Design review of the part shown in the three views and the two pictorial views. Dimensions are in mm from the part's minimum x, y and z. Round coordinates to 2 decimals unless told otherwise and drop trailing zeros. Loops run counter-clockwise (first coordinate to the right, second up) from the corner with the lowest first, then second, coordinate; pieces in that order, holes last.
1. Clearance check with flat-ended pins moving along their axes: pin 1 Ø0.7 at (y, z) = (31.5, 1) entering from -X; pin 2 Ø1.2 at (x, z) = (9.5, 0.5) entering from +Y; pin 3 Ø0.7 at (y, z) = (33, 1.5) entering from +X. State where each tip first meets the part, or that it passes through.
2. To check wall thickness, follow line 1 along X through (y, z) = (32.2, 0.75); line 2 along Y through (x, z) = (19.7, 1); line 3 along X through (y, z) = (27, 1.4). State the ranges of each line that lie inside material, in increasing order.
3. Consider section D-D on x = 6. State the section outline as (y, z) points, then the cut area to 3 significant figures.
4. Consider section B-B on y = 32.2. State the section outline as (x, z) points, then the cut area to 3 significant figures.
5. Consider section C-C on x = 19.7. State the section outline as (y, z) points.
6. Consider section A-A on z = 1.6. State the section outline as (x, y) points.
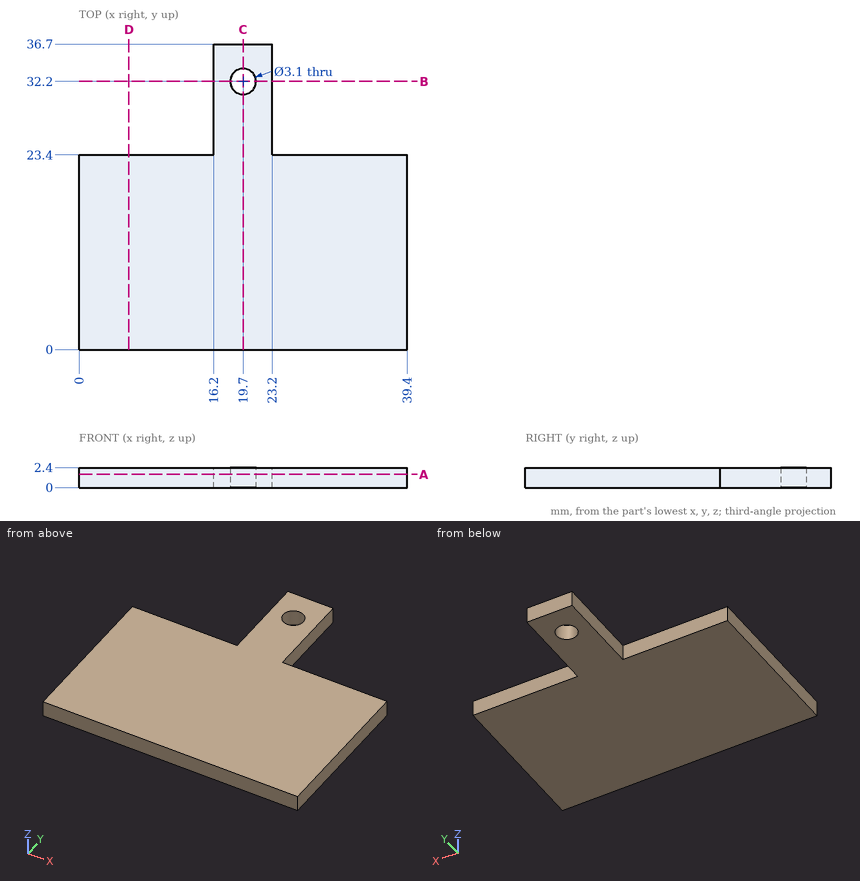
Resolved:
1. pin 1: stops at x = 16.2
1. pin 2: stops at y = 23.4
1. pin 3: stops at x = 23.2
2. line 1: x = 16.2 to 18.15, 21.25 to 23.2
2. line 2: y = 0 to 30.65, 33.75 to 36.7
2. line 3: x = 16.2 to 23.2
3. outline: (0, 0) - (23.4, 0) - (23.4, 2.4) - (0, 2.4) - close
3. area: 56.2 mm2
4. outline: (16.2, 0) - (18.15, 0) - (18.15, 2.4) - (16.2, 2.4) - close; (21.25, 0) - (23.2, 0) - (23.2, 2.4) - (21.25, 2.4) - close
4. area: 9.36 mm2
5. outline: (0, 0) - (30.65, 0) - (30.65, 2.4) - (0, 2.4) - close; (33.75, 0) - (36.7, 0) - (36.7, 2.4) - (33.75, 2.4) - close
6. outline: (0, 0) - (39.4, 0) - (39.4, 23.4) - (23.2, 23.4) - (23.2, 36.7) - (16.2, 36.7) - (16.2, 23.4) - (0, 23.4) - close; hole circle Ø3.1 at (19.7, 32.2)
